```python
from build123d import *

# Parameters (mm, degrees)
SKETCH1_W           = 228.6
SKETCH1_H           = 76.2
SKETCH1_R           = 3.048
SKETCH1_R_2         = 5.08
BOSS_EXTRUDE1_DEPTH = 3.175
SKETCH2_W           = 12.7
SKETCH2_H           = 3.175
BOSS_EXTRUDE2_DEPTH = 3.175
SKETCH3_W           = 22.86
SKETCH3_H           = 25.4
CUT_EXTRUDE1_DEPTH  = 4.175
SKETCH4_W           = 3.175
SKETCH4_H           = 12.7
BOSS_EXTRUDE3_DEPTH = 3.175
SKETCH6_R           = 2.25
CUT_EXTRUDE2_DEPTH  = 4.175
CUT_EXTRUDE3_DEPTH  = 4.175
SKETCH12_W          = 3.175
SKETCH12_H          = 6.35
CUT_EXTRUDE5_DEPTH  = 3.175
SKETCH13_W          = 3.175
SKETCH13_H          = 11.610512243
SKETCH13_H_2        = 11.610512242
BOSS_EXTRUDE5_DEPTH = 3.175


with BuildPart() as part:
    # Sketch1 → Boss-Extrude1 (new body)
    with BuildSketch(Plane.XY):
        with Locations((114.3, 38.1)):
            Rectangle(SKETCH1_W, SKETCH1_H)
        with Locations((215.9, 30.48)):
            Circle(SKETCH1_R, mode=Mode.SUBTRACT)
        with Locations((92.075, 30.48)):
            Circle(SKETCH1_R, mode=Mode.SUBTRACT)
        with Locations((41.56075, 30.48)):
            Circle(SKETCH1_R_2, mode=Mode.SUBTRACT)
    extrude(amount=BOSS_EXTRUDE1_DEPTH)

    # Sketch2 → Boss-Extrude2 (add)
    with BuildSketch(Plane.XZ):
        with Locations((222.25, 1.5875)):
            Rectangle(SKETCH2_W, SKETCH2_H)
        with Locations((196.85, 1.5875)):
            Rectangle(SKETCH2_W, SKETCH2_H)
        with Locations((171.45, 1.5875)):
            Rectangle(SKETCH2_W, SKETCH2_H)
        with Locations((146.05, 1.5875)):
            Rectangle(SKETCH2_W, SKETCH2_H)
        with Locations((120.65, 1.5875)):
            Rectangle(SKETCH2_W, SKETCH2_H)
        with Locations((95.25, 1.5875)):
            Rectangle(SKETCH2_W, SKETCH2_H)
        with Locations((69.85, 1.5875)):
            Rectangle(SKETCH2_W, SKETCH2_H)
        with Locations((44.45, 1.5875)):
            Rectangle(SKETCH2_W, SKETCH2_H)
    extrude(amount=BOSS_EXTRUDE2_DEPTH)

    # Sketch3 → Cut-Extrude1 (cut, through all)
    with BuildSketch(Plane(origin=(0, 0, 0), x_dir=(-1, 0, 0), z_dir=(0, 0, -1))):
        with Locations((-11.43, 12.7)):
            Rectangle(SKETCH3_W, SKETCH3_H)
    extrude(amount=-CUT_EXTRUDE1_DEPTH, mode=Mode.SUBTRACT)

    # Sketch4 → Boss-Extrude3 (add)
    with BuildSketch(Plane.ZY.offset(-22.86)):
        with Locations((1.5875, 6.35)):
            Rectangle(SKETCH4_W, SKETCH4_H)
    extrude(amount=BOSS_EXTRUDE3_DEPTH)

    # Sketch6 → Cut-Extrude2 (cut, through all)
    with BuildSketch(Plane(origin=(0, 0, 0), x_dir=(-1, 0, 0), z_dir=(0, 0, -1))):
        with Locations((-27.16075, 35.48)):
            Circle(SKETCH6_R)
        with Locations((-27.16075, 25.48)):
            Circle(SKETCH6_R)
        with Locations((-76.66075, 35.48)):
            Circle(SKETCH6_R)
        with Locations((-76.66075, 25.48)):
            Circle(SKETCH6_R)
    extrude(amount=-CUT_EXTRUDE2_DEPTH, mode=Mode.SUBTRACT)

    # Sketch8 → Cut-Extrude3 (cut, through all)
    with BuildSketch(Plane.XY.offset(3.175)):
        Polygon((25.4, 76.2), (0, 76.2), (0, 50.8), align=None)
    extrude(amount=-CUT_EXTRUDE3_DEPTH, mode=Mode.SUBTRACT)

    # Sketch12 → Cut-Extrude5 (cut)
    with BuildSketch(Plane(origin=(0, 0, 0), x_dir=(-1, 0, 0), z_dir=(0, 0, -1))):
        with Locations((-220.6625, 66.675)):
            Rectangle(SKETCH12_W, SKETCH12_H)
        with Locations((-174.9425, 66.675)):
            Rectangle(SKETCH12_W, SKETCH12_H)
        with Locations((-129.2225, 66.675)):
            Rectangle(SKETCH12_W, SKETCH12_H)
        with Locations((-83.5025, 66.675)):
            Rectangle(SKETCH12_W, SKETCH12_H)
        with Locations((-37.7825, 66.675)):
            Rectangle(SKETCH12_W, SKETCH12_H)
    extrude(amount=-CUT_EXTRUDE5_DEPTH, mode=Mode.SUBTRACT)

    # Sketch13 → Boss-Extrude5 (add)
    with BuildSketch(Plane(origin=(-25.4, 25.4, 0), x_dir=(0, 0, 1), z_dir=(-0.707106781, 0.707106781, 0))):
        with Locations((1.5875, 66.036792848)):
            Rectangle(SKETCH13_W, SKETCH13_H)
        with Locations((1.5875, 41.726280605)):
            Rectangle(SKETCH13_W, SKETCH13_H_2)
    extrude(amount=BOSS_EXTRUDE5_DEPTH)


solid = part.part
```
Build history of the part. All positions in model axes, mm. A direction names the side the tool comes from. Round coordinates to 2 decimals unless told otherwise and drop trailing zeros. Write each loop counter-clockwise with the first axis right and the second up, starting at its lowest first coordinate (ties: lowest second). Pieces come first, ordered by that corner, then holes.
1) 3-axis set-ups, long thin cutter, end or side, ignore diameter. For faces 1 (the flat face through (125, 35, 0)), 2 (the flat face through (12.6, 63.4, 1.6)): which of +Z, -Z, +X, -X, +Y, -Y reach the whole face in a straight line?
2) Band-saw the part on B-B, the plane x = 106. List the corners of the cut face in (y, z) (3 decimals).
3) Pin check, flat tips, straight feed: pin 1 (1.6 mm diameter, centred on y = -2, z = 1, fed in from -X); pin 2 (1 mm diameter, centred on y = 67.5, z = 2.5, fed in from -X); pin 3 (1.6 mm diameter, centred on x = 107.5, z = 2.5, fed in from +Y). Stop position of each tip, or through.
4) Drill centre lines: probe 1 along X at (y, z) = (30.5, 0.5); probe 2 along X at (y, z) = (75, 2.95); probe 3 along X at (y, z) = (28, 2.55). Where is each one in solid material? Low to high.
5) Band-saw the part on C-C, the plane z = 1.15. Give the number of separate pieces and of enclosed holes in the cut face, and give its area (3 significant figures).
6) Band-saw the part on A-A, the plane y = 30.48. List the corners of the cut face in (x, z) (3 decimals), and give its area (3 significant figures).
7) Mould opens along X. For faces 3 (the cylindrical face through (218.716, 29.313, 1.565)), 4 (the flat face through (19.11, 74.4, 1.57)), 5 (the flat face through (125, 35, 3.175)) say: +X half, -X half, draft (parallel to the pull), parting line (faces both ways), or undercut.
Ans:
1. face 1: -Z, +X, -X, +Y, -Y
1. face 2: +Z, -Z
2. outline: (0, 0) - (76.2, 0) - (76.2, 3.175) - (0, 3.175) - close
3. pin 1: stops at x = 38.1
3. pin 2: stops at x = 16.2
3. pin 3: stops at y = 76.2
4. probe 1: x = 0 to 36.48, 46.64 to 89.03, 95.12 to 212.85, 218.95 to 228.6
4. probe 2: x = 19.71 to 228.6
4. probe 3: x = 0 to 37.13, 45.99 to 90.3, 93.85 to 214.13, 217.67 to 228.6
5. separate pieces: 1
5. enclosed holes: 12
5. area: 16,600 mm2
6. outline: (0, 0) - (36.481, 0) - (36.481, 3.175) - (0, 3.175) - close; (46.641, 0) - (89.027, 0) - (89.027, 3.175) - (46.641, 3.175) - close; (95.123, 0) - (212.852, 0) - (212.852, 3.175) - (95.123, 3.175) - close; (218.948, 0) - (228.6, 0) - (228.6, 3.175) - (218.948, 3.175) - close
6. area: 655 mm2
7. face 3: undercut
7. face 4: -X half
7. face 5: draft
